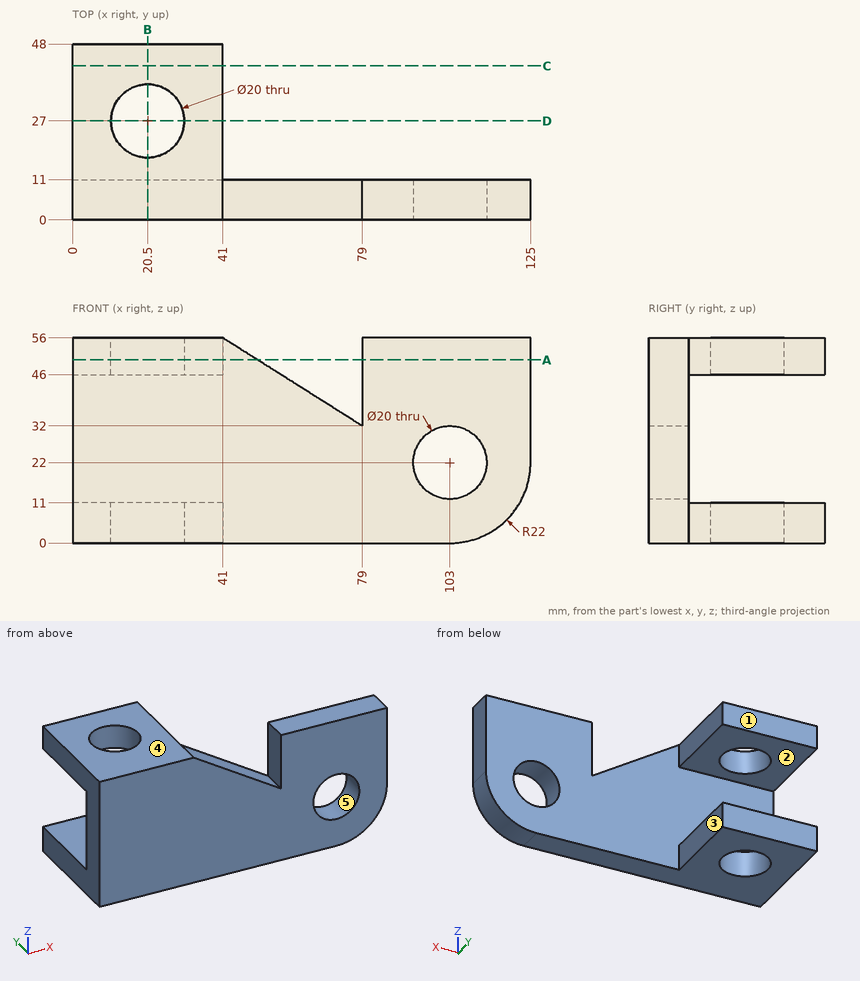
Drawing for the job (mm, zero at the part's lowest x, y, z). A direction names the side the tool comes from. Give positions to 0.01 mm unless a question says otherwise; leave off trailing zeros. Order: outer loops, then holes, each group sorted by start corner. A loop starts at its lowest first (then second) coordinate and runs counter-clockwise, first axis right, second up. Notation, with made-up numbers: M 14.5,85.5 L 20.5,85.5 A9 ccw 20.5,91.5 Z; hole C 12.25,0.5 d9. An arc over 180 degrees is marked long. Put each result on its own line as item: value. Start each with the question number.
(1) Mould opens along Z. For the marked faces 3, 4 and 5 say: +Z half, -Z half, draft (parallel to the pull), parting line (faces both ways), or undercut.
(2) Saw through at B-B, the plane x = 20.5. Write the cut outline in (y, z), then the cut area to 3 significant figures.
(3) Saw through at C-C, the plane y = 42. Write the cut outline in (x, z).
(4) Saw through at A-A, the plane z = 50. Write the cut outline in (x, y).
(5) Flat gauge pins, fed straight in: pin 1 Ø18 at (x, y) = (20.5, 27) entering from -Z (3 decimals); pin 2 Ø10 at (x, z) = (91.5, 28) entering from +Y; pin 3 Ø11 at (y, z) = (37.5, 53) entering from +X. Where does each tip first touch, or does it go through?
(6) Which spindle directions (+Z, -Z, +X, -X, +Y, -Y) get a long thin tool onto all of the face, cutting with end or side? Do the marked faces 1 and 2. Say none if no direction does.
(7) Drill centre lines: line 1 along X through (y, z) = (6.5, 22); line 2 along Y through (x, z) = (20, 50); line 3 along Z through (x, y) = (39.5, 39). Where is each one in solid material? Low to high.
(8) Saw through at D-D, the plane y = 27. Write the cut outline in (x, z).
Check result:
1. face 3: draft
1. face 4: +Z half
1. face 5: undercut
2. outline: M 0,0 L 17,0 L 17,11 L 11,11 L 11,46 L 17,46 L 17,56 L 0,56 Z; M 37,0 L 48,0 L 48,11 L 37,11 Z; M 37,46 L 48,46 L 48,56 L 37,56 Z
2. area: 973 mm2
3. outline: M 0,0 L 41,0 L 41,11 L 0,11 Z; M 0,46 L 41,46 L 41,56 L 0,56 Z
4. outline: M 0,0 L 50.5,0 L 50.5,11 L 41,11 L 41,48 L 0,48 Z; M 79,0 L 125,0 L 125,11 L 79,11 Z; hole C 20.5,27 d20
5. pin 1: passes through
5. pin 2: stops at y = 11
5. pin 3: stops at x = 41
6. face 1: +Z, -Z, +X, -X, +Y
6. face 2: +X, -X, +Y
7. line 1: x = 0 to 93, 113 to 125
7. line 2: y = 0 to 17.01, 36.99 to 48
7. line 3: z = 0 to 11, 46 to 56
8. outline: M 0,0 L 10.5,0 L 10.5,11 L 0,11 Z; M 0,46 L 10.5,46 L 10.5,56 L 0,56 Z; M 30.5,0 L 41,0 L 41,11 L 30.5,11 Z; M 30.5,46 L 41,46 L 41,56 L 30.5,56 Z
